Can you work these out from the model? Positions are in its coordinate system, mm. A direction names the side the tool comes from. Coordinates: 2 decimals unless noted, no trailing zeros. Write each loop counter-clockwise with the first axis right and the second up, starting at its lowest first coordinate (ties: lowest second). Pieces come first, ordered by that corner, then holes. Notation, with made-up numbers: (56.5, -21) - (99.5, -21) arc R18 ccw to (99.5, 11) - close; hole circle Ø10 at (-16.75, 12). An arc over 180 degrees is marked (long way). Write each question's results on one line, items separated by ' | '. Start each with the question number.
```python
from build123d import *

# Parameters (mm, degrees)
SKETCH1_W           = 90
SKETCH1_H           = 110
BOSS_EXTRUDE1_DEPTH = 82
CUT_EXTRUDE1_DEPTH  = 80
BOSS_EXTRUDE2_DEPTH = 40
CUT_EXTRUDE2_DEPTH  = 40
SKETCH11_R          = 12
CUT_EXTRUDE3_DEPTH  = 94
SKETCH12_R          = 12.003282012
CUT_EXTRUDE4_DEPTH  = 113


with BuildPart() as part:
    # Sketch1 → Boss-Extrude1 (new body)
    with BuildSketch(Plane(origin=(0, 0, 0), x_dir=(1, 0, 0), z_dir=(0, 1, 0))):
        with Locations((-14.558423382, 3.303288505)):
            Rectangle(SKETCH1_W, SKETCH1_H)
    extrude(amount=BOSS_EXTRUDE1_DEPTH)

    # 3DSketch1 → Cut-Extrude1 (cut)
    with BuildSketch(Plane(origin=(28.441576618, 82, 49.696711495), x_dir=(-0.6300408568675958, 0, -0.7765619863716906), z_dir=(0, 1, 0))):
        Polygon((0, 0), (82.315570555, -66.784330828), (136.499084246, 0), (54.183513691, 66.784330828), align=None)
    extrude(amount=-CUT_EXTRUDE1_DEPTH, mode=Mode.SUBTRACT)

    # Sketch7 → Boss-Extrude2 (add)
    with BuildSketch(Plane.XZ):
        Polygon((30.441576618, 26.660546429), (30.441576618, -33.267123439), (10.560534859, -58.303288505), (-39.439465141, -58.303288505), (-59.558423382, -33.267123439), (-59.558423382, 26.660546429), (-39.439465141, 51.696711495), (10.322618378, 51.696711495), align=None)
    extrude(amount=BOSS_EXTRUDE2_DEPTH)

    # Sketch10 → Cut-Extrude2 (cut)
    with BuildSketch(Plane(origin=(0, 2, 0), x_dir=(1, 0, 0), z_dir=(0, 1, 0))):
        Polygon((28.441576618, -25.9565253), (28.441576618, 32.569615498), (9.594834599, 56.303288505), (-38.480908378, 56.303288505), (-57.558423382, 32.563102309), (-57.558423382, -25.9565253), (-38.480908378, -49.696711495), (9.364061615, -49.696711495), align=None)
    extrude(amount=-CUT_EXTRUDE2_DEPTH, mode=Mode.SUBTRACT)

    # Sketch11 → Cut-Extrude3 (cut)
    with BuildSketch(Plane(origin=(30.441576618, 0, 0), x_dir=(0, 0, -1), z_dir=(1, 0, 0))):
        with Locations((3.303288505, -20)):
            Circle(SKETCH11_R)
    extrude(amount=-CUT_EXTRUDE3_DEPTH, mode=Mode.SUBTRACT)

    # Sketch12 → Cut-Extrude4 (cut)
    with BuildSketch(Plane.XY.offset(51.696711495)):
        with Locations((-14.558423382, -20)):
            Circle(SKETCH12_R)
    extrude(amount=-CUT_EXTRUDE4_DEPTH, mode=Mode.SUBTRACT)


solid = part.part
```
Q1. If we section it at C-C (z = -12): Please give me the cut outline in (x, y).
Q2. I'm going to push flat-ended pins straight in: pin 1 Ø3 at (x, z) = (-41, 4.5) entering from +Y; pin 2 Ø9.5 at (x, z) = (-50, -44.5) entering from +Y; pin 3 Ø21.5 at (x, y) = (-14.56, -20) entering from +Z. Where does each tip first touch, or does it pass through?
Q3. If we section it at B-B (x = -14.5): Please give me the cut outline in (y, z), then the cut area to 3 significant figures.
Q4. Thinking about a two-plate mould opening in X: for faces 1 (the face through (-52, 0, -49)), 2 (the face through (-59.558, 34, -3)), 3 (the face through (-23.41, -11.89, -57.29)), which applies, pulls with the +X half, pulls with the -X half, needs draft (parallel to the pull), parting line crosses it, or undercut?
Q5. For faces 4 (the face through (20.241, -19.72, 39.354)), 5 (the face through (-49.36, -19.72, -45.96)), 6 (the face through (-15, -38, -4)), 7 (the face through (-49.64, -19.72, 39)), which set-ups out of +Z, -Z, +X, -X, +Y, -Y let a thin tool reach every point of the face, with its end or its side?
Q6. If we section it at A-A (y = -20): Count the separate pieces of the cut face and the enclosed holes in it, then the cut area to 3 significant figures.
Q7. I need wall thicknesses on line 1 along Z through (x, y) = (-29, 16.5); line 2 along X through (y, z) = (6, -37); line 3 along Y through (x, z) = (-13.5, -36.5). Which ranges of each line are inside material? Lowest first, please. Write a range as from..to.
Q8. If we section it at D-D (y = 36.5): Please give me the cut outline in (x, z).
Answer list:
1) outline: (-59.56, -40) - (30.44, -40) - (30.44, -28.27) - (28.44, -28.27) - (28.44, -38) - (-57.56, -38) - (-57.56, -28.27) - (-59.56, -28.27) - close; (-59.56, -11.73) - (-57.56, -11.73) - (-57.56, 82) - (-59.56, 82) - close; (28.44, -11.73) - (30.44, -11.73) - (30.44, 82) - (28.44, 82) - close
2) pin 1: stops at y = -38 | pin 2: stops at y = 2 | pin 3: passes through
3) outline: (-40, -58.3) - (-32, -58.3) - (-32, -56.3) - (-38, -56.3) - (-38, 49.7) - (-32, 49.7) - (-32, 51.7) - (-40, 51.7) - close; (-8, -58.3) - (82, -58.3) - (82, -56.3) - (-8, -56.3) - close; (-8, 49.7) - (82, 49.7) - (82, 51.7) - (-8, 51.7) - close | area: 604 mm2
4) face 1: needs draft | face 2: pulls with the -X half | face 3: undercut
5) face 4: +Z, +X, -Y | face 5: -Z, -X, -Y | face 6: +Y | face 7: +Z, -X, -Y
6) separate pieces: 4 | enclosed holes: 0 | area: 491 mm2
7) line 1: z = -58.3..-56.3, 49.7..51.7 | line 2: x = -59.56..-57.56, 28.44..30.44 | line 3: y = -40..-38
8) outline: (-59.56, -58.3) - (30.44, -58.3) - (30.44, 51.7) - (-59.56, 51.7) - close; hole (-57.56, -56.3) - (28.44, -56.3) - (28.44, 49.7) - (-57.56, 49.7) - close
